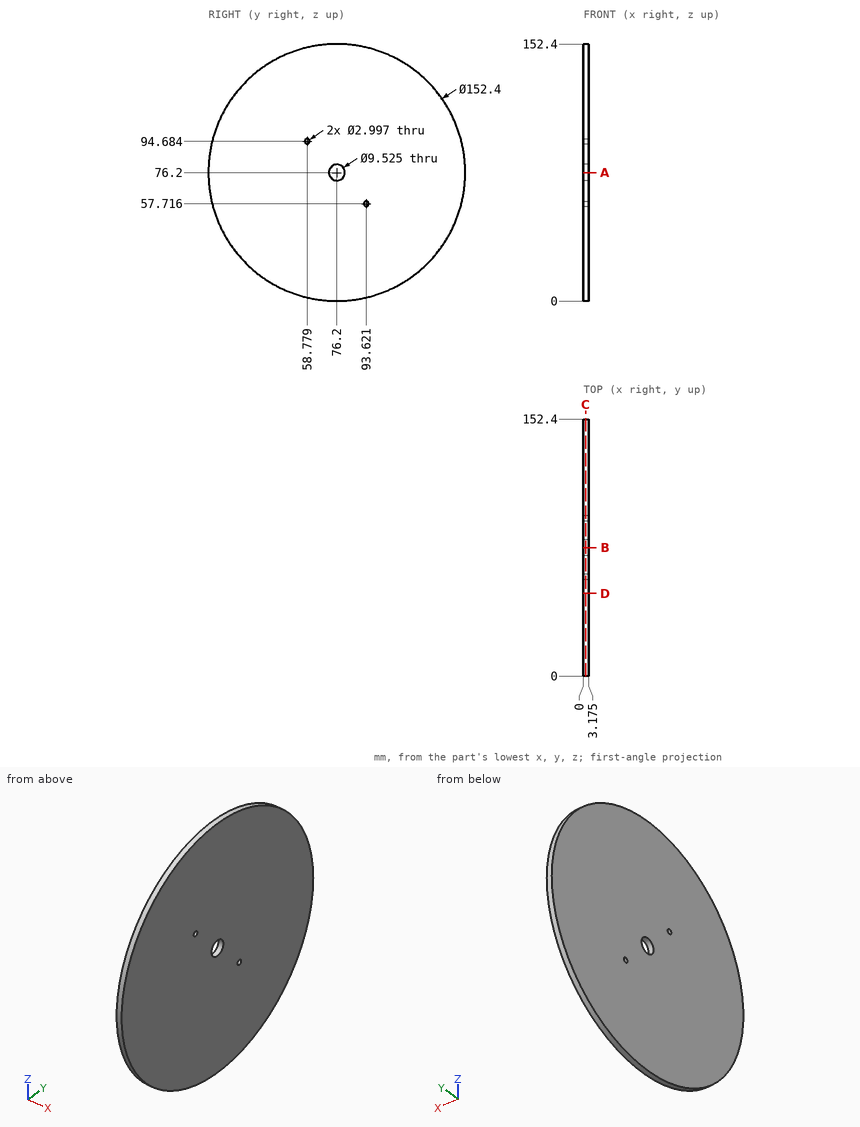
Answer from the drawing. Dimensions are ordinates in mm from the lowest x, y and z of the part. Round coordinates to 2 decimals unless told otherwise and drop trailing zeros. Write each loop counter-clockwise with the first axis right and the second up, starting at its lowest first coordinate (ties: lowest second). Pieces come first, ordered by that corner, then holes. Notation, with made-up numbers: (43, 46.5) - (94, 46.5) arc R26 ccw to (94, 84.5) - close; hole circle Ø3 at (-2, 41.25). An arc over 180 degrees is marked (long way). Use a Markdown table: item, result.
(1) This flat-tipped pin is pushed along its axis until it touches: pin 1 Ø2.5 at (y, z) = (58.78, 94.68) entering from +X. Where does it stop, or does it pass through?
Reported:
| item | result |
|---|---|
| pin 1 | through |
(2) The part is cut by section A-A (z = 76.2). Write down the section's boundary in (x, y) (1 decimal).
Reported:
| item | result |
|---|---|
| outline | (0, 0) - (3.2, 0) - (3.2, 71.4) - (0, 71.4) - close; (0, 81) - (3.2, 81) - (3.2, 152.4) - (0, 152.4) - close |
(3) Straight lines are drawn through the part: line 1 along Z through (x, y) = (1.1, 76.2); line 2 along Y through (x, z) = (0.7, 94) (1 decimal). For each, find the intervals that lie inside material, in ascending order. Write a range as [from, to].
Reported:
| item | result |
|---|---|
| line 1 | [0, 71.44], [80.96, 152.4] |
| line 2 | [2.1, 57.4], [60.1, 150.3] |
(4) The part is cut by section C-C (x = 1.4). Write down the section's boundary in (y, z) (1 decimal).
Reported:
| item | result |
|---|---|
| outline | circle Ø152.4 at (76.2, 76.2); hole circle Ø3 at (58.8, 94.7); hole circle Ø9.5 at (76.2, 76.2); hole circle Ø3 at (93.6, 57.7) |
(5) The part is cut by section D-D (y = 49). Write down the section's boundary in (x, z) (1 decimal), then the cut area to 3 significant figures.
Reported:
| item | result |
|---|---|
| outline | (0, 5) - (3.2, 5) - (3.2, 147.4) - (0, 147.4) - close |
| area | 452 mm2 |
